Can you work these out from the drawing? Everything is in mm from the part's minimum corner. A direction names the side the tool comes from. Give positions to 0.01 mm unless a question says otherwise; leave off trailing zeros. Order: outer loops, then holes, each group sorted by start corner. A loop starts at its lowest first (then second) coordinate and runs counter-clockwise, first axis right, second up. Notation, with made-up numbers: M 71,30 L 107,30 A11 cw 107,41 Z; hole C 74.5,78.5 d4. An arc over 180 degrees is marked long. Answer in a Markdown table with one row per item. Add a question column.
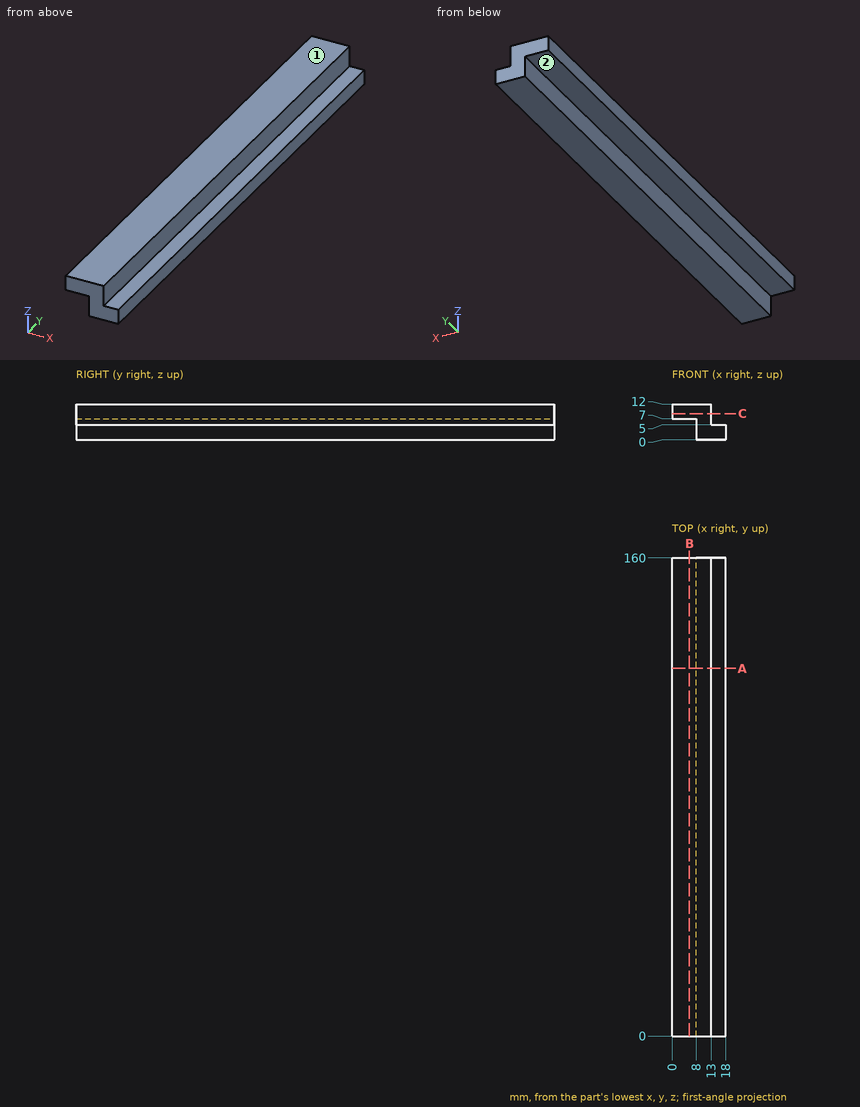
1. If I drill on line 1 along X through (y, z) = (136, 2.75); line 2 along Z through (x, y) = (4.5, 21); line 3 along X through (y, z) = (102.5, 9.5), over which ranges is the centre line in solid material (lowest first)? Write a range as [from, to].
2. Suppose I cut it at B-B on x = 5.75. List the corners of the cut face in (y, z) for me.
3. For the marked faces 1 and 2, which set-ups out of +Z, -Z, +X, -X, +Y, -Y let a thin tool reach every point of the face, with its end or its side?
4. Suppose I cut it at A-A on y = 123. List the corners of the cut face in (x, z) for me, plus the area to 3 significant figures.
5. Will these pins go through, and if not, where does the flat tip stop? P1, Ø1.5, axis at y = 101, z = 8, coming from the +X side; P2, Ø5, axis at x = 15, y = 110, coming from the +Z side; P3, Ø3, axis at x = 3.5, y = 95.5, coming from the -Z side.
6. Suppose I cut it at C-C on z = 8.75. List the corners of the cut face in (x, y) for me, plus the area to 3 significant figures.
Findings below:
| question | item | result |
|---|---|---|
| 1 | line 1 | [8, 18] |
| 1 | line 2 | [7, 12] |
| 1 | line 3 | [0, 13] |
| 2 | outline | M 0,7 L 160,7 L 160,12 L 0,12 Z |
| 3 | face 1 | +Z, +X, -X, +Y, -Y |
| 3 | face 2 | -Z, -X, +Y, -Y |
| 4 | outline | M 0,7 L 8,7 L 8,0 L 18,0 L 18,5 L 13,5 L 13,12 L 0,12 Z |
| 4 | area | 125 mm2 |
| 5 | P1 | x = 13 |
| 5 | P2 | z = 12 |
| 5 | P3 | z = 7 |
| 6 | outline | M 0,0 L 13,0 L 13,160 L 0,160 Z |
| 6 | area | 2,080 mm2 |
